Input: part model. Units: mm. Frame: model coordinates. Face numbers are marked on the shaded views. Give positions to 0.01 mm unless a question says otherwise; leave off trailing zeros. Loops run counter-clockwise (first coordinate to the right, second up) from the corner with the lowest first, then second, coordinate; pieces in that order, holes last. Notation, with made-up numbers: M -6,84.5 L 35,84.5 A22 ccw 35,108.5 Z; hole C -40,44 d11. An arc over 180 degrees is marked long. Use CSV: the item, a comma, the result in double quotes. Start each with the question number.
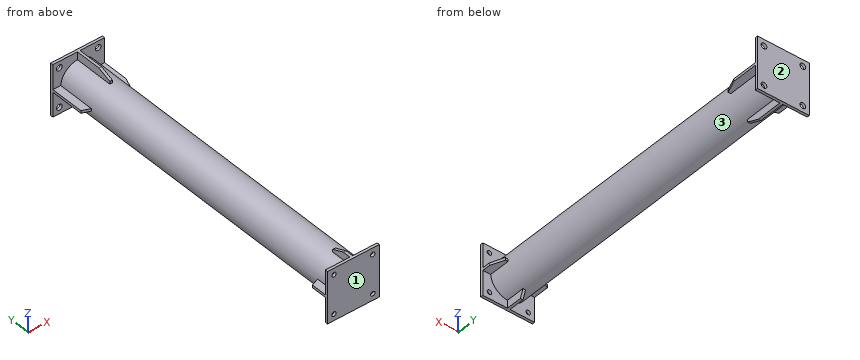
from build123d import *

# Parameters (mm, degrees)
F0_R          = 70
F0_R_2        = 65
F1_DEPTH      = 1264
F2_W          = 200
F2_H          = 200
F2_R          = 11
F3_DEPTH      = 10
F4_W          = 30.1787997812
F4_H          = 10
F4_W_2        = 10
F4_H_2        = 30.1787997812
F5_DEPTH      = 150
F6_T1_DEPTH   = 269.311363913
F6_T3_DEPTH   = 269.311363913
F6_T8_DEPTH   = 269.311363913
F6_S9_R       = 70
F6_T10_DEPTH  = 139
F8_W          = 200
F8_H          = 200
F8_R          = 8.5
F9_DEPTH      = 10
F10_W         = 10
F10_H         = 30.1787997812
F10_W_2       = 30.1787997812
F10_H_2       = 10
F11_DEPTH     = 80
F12_T1_DEPTH  = 269.311363913
F12_T3_DEPTH  = 269.311363913
F12_T8_DEPTH  = 269.311363913
F12_S9_R      = 70
F12_T10_DEPTH = 139
F12_T14_DEPTH = 269.311363913
F12_S15_R     = 70
F12_T16_DEPTH = 139


# Not quite as in the source:
# - a fillet or chamfer that OpenCascade refuses, or shapes differently, is made with other operations: its cross-section is extruded or revolved along the edge and cut away or added


with BuildPart() as f1:
    # F0 (on Front) → F1 (new body)
    with BuildSketch(Plane.XZ):
        Circle(F0_R)
        Circle(F0_R_2, mode=Mode.SUBTRACT)
    extrude(amount=F1_DEPTH)

    # F2 (on Front) → F3 (join)
    with BuildSketch(Plane.XZ):
        Rectangle(F2_W, F2_H)
        with Locations((-75, -75)):
            Circle(F2_R, mode=Mode.SUBTRACT)
        with Locations((75, -75)):
            Circle(F2_R, mode=Mode.SUBTRACT)
        with Locations((-75, 75)):
            Circle(F2_R, mode=Mode.SUBTRACT)
        with Locations((75, 75)):
            Circle(F2_R, mode=Mode.SUBTRACT)
    extrude(amount=-F3_DEPTH)

    # F4 (on Front) → F5 (join)
    with BuildSketch(Plane.XZ):
        with Locations((-84.9106001094, 0)):
            Rectangle(F4_W, F4_H)
        with Locations((0, 84.9106001094)):
            Rectangle(F4_W_2, F4_H_2)
        with Locations((84.9106001094, 0)):
            Rectangle(F4_W, F4_H)
        with Locations((0, -84.9106001094)):
            Rectangle(F4_W_2, F4_H_2)
    extrude(amount=F5_DEPTH)

    # F6: chamfer of 50 x 20 on 4 edges, made by hand

    # F6_s2 → F6_t1 (cut)
    with BuildSketch(Plane.YZ.offset(-134.6556819565)):
        Polygon((-100, 100), (-150, 80), (-150, 100), align=None)
        Polygon((-100, -100), (-150, -80), (-150, -100), align=None)
    extrude(amount=F6_T1_DEPTH, mode=Mode.SUBTRACT)

    # F6_s4 → F6_t3 (cut)
    with BuildSketch(Plane.XY.offset(-134.6556819565)):
        Polygon((100, -100), (80, -150), (100, -150), align=None)
    extrude(amount=F6_T3_DEPTH, mode=Mode.SUBTRACT)


with BuildPart() as f6_tool6:
    # F6_s7 → F6_t8 (new body)
    with BuildSketch(Plane.XY.offset(134.6556819565)):
        Polygon((-100, -130), (-50, -150), (-100, -150), align=None)
    extrude(amount=-F6_T8_DEPTH)

    # F6_s9 → F6_t10 (cut, symmetric)
    with BuildSketch(Plane.XZ.offset(140)):
        Circle(F6_S9_R)
    extrude(amount=F6_T10_DEPTH, both=True, mode=Mode.SUBTRACT)


with BuildPart() as f1_1:
    add(f1.part)

    # F6_t5: cut F6_tool6
    add(f6_tool6.part, mode=Mode.SUBTRACT)

    # F8 (on offset) → F9 (join)
    with BuildSketch(Plane.XZ.offset(1264)):
        Rectangle(F8_W, F8_H)
        with Locations((-75, -75)):
            Circle(F8_R, mode=Mode.SUBTRACT)
        with Locations((75, -75)):
            Circle(F8_R, mode=Mode.SUBTRACT)
        with Locations((-75, 75)):
            Circle(F8_R, mode=Mode.SUBTRACT)
        with Locations((75, 75)):
            Circle(F8_R, mode=Mode.SUBTRACT)
    extrude(amount=F9_DEPTH)

    # F10 (on face) → F11 (join)
    with BuildSketch(Plane(origin=(0, -1264, 0), x_dir=(-1, 0, 0), z_dir=(0, 1, 0))):
        with Locations((0, 84.9106001094)):
            Rectangle(F10_W, F10_H)
        with Locations((84.9106001094, 0)):
            Rectangle(F10_W_2, F10_H_2)
        with Locations((0, -84.9106001094)):
            Rectangle(F10_W, F10_H)
        with Locations((-84.9106001094, 0)):
            Rectangle(F10_W_2, F10_H_2)
    extrude(amount=F11_DEPTH)

    # F12: chamfer of 20 x 50 on 4 edges, made by hand

    # F12_s2 → F12_t1 (cut)
    with BuildSketch(Plane.YZ.offset(-134.6556819565)):
        Polygon((-1234, 100), (-1184, 80), (-1184, 100), align=None)
    extrude(amount=F12_T1_DEPTH, mode=Mode.SUBTRACT)

    # F12_s4 → F12_t3 (cut)
    with BuildSketch(Plane.XY.offset(-134.6556819565)):
        Polygon((100, -1234), (80, -1184), (100, -1184), align=None)
    extrude(amount=F12_T3_DEPTH, mode=Mode.SUBTRACT)


with BuildPart() as f12_tool6:
    # F12_s7 → F12_t8 (new body)
    with BuildSketch(Plane.XY.offset(-134.6556819565)):
        Polygon((-100, -1204), (-50, -1184), (-100, -1184), align=None)
    extrude(amount=F12_T8_DEPTH)

    # F12_s9 → F12_t10 (cut, symmetric)
    with BuildSketch(Plane.XZ.offset(1194)):
        Circle(F12_S9_R)
    extrude(amount=F12_T10_DEPTH, both=True, mode=Mode.SUBTRACT)


with BuildPart() as f1_2:
    add(f1_1.part)

    # F12_t5: cut F12_tool6
    add(f12_tool6.part, mode=Mode.SUBTRACT)


with BuildPart() as f12_tool12:
    # F12_s13 → F12_t14 (new body)
    with BuildSketch(Plane.YZ.offset(134.6556819565)):
        Polygon((-1204, -100), (-1184, -50), (-1184, -100), align=None)
    extrude(amount=-F12_T14_DEPTH)

    # F12_s15 → F12_t16 (cut, symmetric)
    with BuildSketch(Plane.XZ.offset(1194)):
        Circle(F12_S15_R)
    extrude(amount=F12_T16_DEPTH, both=True, mode=Mode.SUBTRACT)


with BuildPart() as f1_3:
    add(f1_2.part)

    # F12_t11: cut F12_tool12
    add(f12_tool12.part, mode=Mode.SUBTRACT)


solid = f1_3.part
Item 1: Material intervals for line 1 (Z direction, x = 75, y = 6); line 2 (Z direction, x = -75, y = -1269.5); line 3 (Y direction, x = 36, z = -11.5), sorted ascending.
Item 2: Section B-B (y = -784). Output: boundary loops of the cut face in (x, z).
Item 3: Mould query, pull axis Y, two halves, no side actions, for the marked faces 1, 2 and 3. Classes: +Y half, -Y half, draft (parallel to the pull), parting line (faces both ways), or undercut.
Item 4: First-contact query: pin 1 Ø6 at (x, y) = (31, -1124) entering from +Z; pin 2 Ø24 at (y, z) = (-46.5, -88) entering from +X; pin 3 Ø2 at (x, y) = (58, -970.5) entering from +Z; pin 4 Ø19.5 at (x, z) = (-75, -75) entering from -Y. Flat tips, straight axial feed; report the tip coordinate or a pass-through.
Item 5: Section C-C (x = -48). Output: boundary loops of the cut face in (y, z), then the cut area to 3 significant figures.
Item 6: Section A-A (z = -35). Output: boundary loops of the cut face in (x, y), then the cut area to 3 significant figures.
Recorded:
1,line 1,"-100 to -86, -64 to 64, 86 to 100"
1,line 2,"-100 to -83.5, -66.5 to 66.5, 83.5 to 100"
1,line 3,"-1274 to -1264, 0 to 10"
2,outline,"C 0,0 d140; hole C 0,0 d130"
3,face 1,"-Y half"
3,face 2,"+Y half"
3,face 3,"undercut"
4,pin 1,"z = 64.16"
4,pin 2,"x = 5"
4,pin 3,"z = 40.63"
4,pin 4,"y = -1274"
5,outline,"M -1274,-100 L -1264,-100 L -1264,-50.95 L 0,-50.95 L 0,-100 L 10,-100 L 10,100 L 0,100 L 0,50.95 L -1264,50.95 L -1264,100 L -1274,100 Z; hole M -1264,-43.83 L 0,-43.83 L 0,43.83 L -1264,43.83 Z"
5,area,"22,000 mm²"
6,outline,"M -100,-1274 L 100,-1274 L 100,-1264 L 60.62,-1264 L 60.62,0 L 100,0 L 100,10 L -100,10 L -100,0 L -60.62,0 L -60.62,-1264 L -100,-1264 Z; hole M -54.77,-1264 L 54.77,-1264 L 54.77,0 L -54.77,0 Z"
6,area,"18,800 mm²"
